Autodesk Inventor part; units mm, degrees
ref_plane "YZ Plane" through (0, 0, 0) normal (1, 0, 0) x (0, 1, 0)
ref_plane "XZ Plane" through (0, 0, 0) normal (0, 1, 0) x (-1, 0, 0)
ref_plane "XY Plane" through (0, 0, 0) normal (0, 0, 1) x (1, 0, 0)
sketch "Sketch1" plane through (0, 0, 0) normal (0, 0, 1) x (1, 0, 0)
  line L0 (0, 0) -> (50.8, 0)
  line L1 (50.8, 0) -> (50.8, 50.8)
  line L2 (50.8, 50.8) -> (0, 50.8)
  line L3 (0, 50.8) -> (0, 0)
  dimension "d0" = 50.8
  dimension "d1" = 50.8
extrude "Extrusion1" add sketch "Sketch1" along normal blind 3.175
sketch "Sketch2" plane through (0, 0, 3.175) normal (0, 0, 1) x (1, 0, 0)
  line L0 (0, 0) -> (50.8, 0)
  line L1 (50.8, 0) -> (50.8, 50.8)
  line L2 (50.8, 50.8) -> (0, 50.8)
  line L3 (0, 50.8) -> (0, 0)
  point P0 (12.7, 12.7)
  point P1 (38.1, 12.7)
  dimension "d4" = 12.7
  dimension "d5" = 12.7
  dimension "d6" = 12.7
  dimension "d7" = 12.7
hole "Hole1" at (12.7, 12.7, 3.175) at (38.1, 12.7, 3.175) direction (0, 0, -1) diameter 6.35 end through all
sketch "Sketch3" plane through (0, 0, 0) normal (0, 0, -1) x (-1, 0, 0)
  line L0 (0, 0) -> (-50.8, 0)
  line L1 (-50.8, 0) -> (-50.8, 50.8)
  line L2 (-50.8, 0) -> (-50.8, 50.8)
  line L3 (-50.8, 25.4) -> (-38.1, 50.8)
  line L4 (-50.8, 50.8) -> (0, 50.8) construction
  line L5 (-38.1, 50.8) -> (-12.7, 50.8) construction
  line L6 (-12.7, 50.8) -> (0, 25.4)
  line L7 (0, 50.8) -> (0, 0)
  line L8 (-38.1, 50.8) -> (-50.8, 50.8)
  line L9 (-50.8, 50.8) -> (-50.8, 25.4)
  line L10 (-12.7, 50.8) -> (0, 50.8)
  line L11 (0, 50.8) -> (0, 25.4)
  dimension "d19" = 25.4
  dimension "d20" = 25.4
  dimension "d21" = 25.4
  dimension "d22" = 12.7
extrude "Extrusion2" cut sketch "Sketch3" against normal blind 25.4
sketch "Sketch4" plane through (0, 0, 0) normal (0, 0, -1) x (-1, 0, 0)
  line L0 (0, 25.4) -> (-12.7, 50.8)
  line L1 (-38.1, 50.8) -> (-12.7, 50.8)
  line L2 (-38.1, 50.8) -> (-50.8, 25.4)
  line L3 (-50.8, 0) -> (-50.8, 25.4)
  line L4 (0, 0) -> (-50.8, 0)
  line L5 (0, 25.4) -> (0, 0)
  circle A0 centre (-12.7, 12.7) radius 3.175
  circle A1 centre (-38.1, 12.7) radius 3.175
  circle A2 centre (-25.4, 28.575) radius 3.175 construction
  line L6 (-34.925, 50.8) -> (-28.4572, 27.7183)
  line L7 (-15.875, 50.8) -> (-22.3428, 27.7183)
  arc A3 (-28.4572, 27.7183) -> (-22.3428, 27.7183) centre (-25.4, 28.575) ccw
  line L8 (-34.925, 50.8) -> (-15.875, 50.8)
  line L9 (-38.1, 50.8) -> (-12.7, 50.8)
  dimension "d25" = 6.35
  dimension "d26" = 22.225
  dimension "d27" = 12.7
  dimension "d28" = 3.175
  dimension "d29" = 3.175
extrude "Extrusion3" cut sketch "Sketch4" against normal blind 25.4 contours L7 A3 L6 L1
properties part number "pickup arm tab" material "Aluminum 6061"
Design review of the part built by this model. Coordinates are the model's own, in mm. A direction names the side the tool comes from. Round coordinates to 2 decimals unless told otherwise and drop trailing zeros. Write each loop counter-clockwise with the first axis right and the second up, starting at its lowest first coordinate (ties: lowest second). Pieces come first, ordered by that corner, then holes.
Item 1: Consider section A-A on y = 12.7. Give the boundary of the cut face in (x, z) (3 decimals).
Item 2: Draft analysis for pull direction Y (two halves, no side actions). For faces 3 (the flat face through (19.064, 39.421, 1.565)), 4 (the flat face through (50.8, 13, 2)), 5 (the cylindrical face through (35.423, 10.993, 1.565)), state which applies: released by +Y, released by -Y, zero draft, split by the parting line, or undercut.
Item 3: Consider section D-D on x = 48.5. Give the boundary of the cut face in (y, z) (3 decimals), and give its area (4 significant figures).
Item 4: Wall thickness on L1, parallel to X at y = 12.7, z = 0.95 (3 decimals); L2, parallel to X at y = 48, z = 2.35; L3, parallel to X at y = 27, z = 1.1: over which ranges is each line inside the solid? List them lowest first.
Item 5: Consider section B-B on z = 0.85. Give the boundary of the cut face in (x, y) (3 decimals), and give its area (3 significant figures).
Item 6: For faces 1 (the flat face through (14, 50.8, 2)), 2 (the flat face through (31.736, 39.421, 1.565)), list the 3-axis set-ups (+Z, -Z, +X, -X, +Y, -Y) from which the entire face can be reached by the end or side of a thin tool; tool diameter is ignored.
Item 7: Consider section C-C on y = 42. Give the boundary of the cut face in (x, z) (3 decimals), and give its area (3 significant figures).
Check values:
1. outline: (0, 0) - (9.525, 0) - (9.525, 3.175) - (0, 3.175) - close; (15.875, 0) - (34.925, 0) - (34.925, 3.175) - (15.875, 3.175) - close; (41.275, 0) - (50.8, 0) - (50.8, 3.175) - (41.275, 3.175) - close
2. face 3: released by +Y
2. face 4: zero draft
2. face 5: undercut
3. outline: (0, 0) - (30, 0) - (30, 3.175) - (0, 3.175) - close
3. area: 95.25 mm2
4. L1: x = 0 to 9.525, 15.875 to 34.925, 41.275 to 50.8
4. L2: x = 11.3 to 16.66, 34.14 to 39.5
4. L3: x = 0.8 to 22.64, 28.16 to 50
5. outline: (0, 0) - (50.8, 0) - (50.8, 25.4) - (38.1, 50.8) - (34.925, 50.8) - (28.457, 27.718) arc R3.175 cw to (22.343, 27.718) - (15.875, 50.8) - (12.7, 50.8) - (0, 25.4) - close; hole circle Ø6.35 at (12.7, 12.7); hole circle Ø6.35 at (38.1, 12.7)
5. area: 1,890 mm2
6. face 1: +Z, -Z, +X, -X, +Y
6. face 2: +Z, -Z, +Y
7. outline: (8.3, 0) - (18.341, 0) - (18.341, 3.175) - (8.3, 3.175) - close; (32.459, 0) - (42.5, 0) - (42.5, 3.175) - (32.459, 3.175) - close
7. area: 63.8 mm2
